from build123d import *

# Parameters (mm, degrees)
PAD011_DEPTH           = 3.5
POCKET_DEPTH           = 1
SKETCH_W               = 3
SKETCH_H               = 7
POCKET024_DEPTH        = 3.501
LINEARPATTERN001_COUNT = 3
LINEARPATTERN001_PITCH = 20


with BuildPart() as part:
    # Sketch030 (on Face1 of Binder) → Pad011 (new body)
    with BuildSketch(Plane(origin=(0, 0, -1.5), x_dir=(1, 0, 0), z_dir=(0, 0, -1))):
        Polygon((17.648, -218.84), (19.648, -220.84), (105.648, -220.84), (107.648, -218.84), (107.648, -139.715), (105.648, -137.715), (107.648, -135.715), (107.648, -56.59), (105.648, -54.59), (19.648, -54.59), (17.648, -56.59), (17.648, -135.715), (19.648, -137.715), (17.648, -139.715), align=None)
    extrude(amount=-PAD011_DEPTH)

    # Sketch034 (on Face4 of Pad011) → Pocket (cut)
    with BuildSketch(Plane.XY.offset(2)):
        Polygon((19.523, 137.84), (62.523, 137.84), (62.523, 220.84), (62.773, 220.84), (62.773, 137.84), (105.773, 137.84), (105.773, 137.59), (62.773, 137.59), (62.773, 54.59), (62.523, 54.59), (62.523, 137.59), (19.523, 137.59), align=None)
    extrude(amount=-POCKET_DEPTH, mode=Mode.SUBTRACT)

    # Sketch (on Face4 of Clone001) → Pocket024 (cut, through all)
    with BuildSketch(Plane.XY.offset(2)):
        with Locations((42.648, 137.715)):
            Rectangle(SKETCH_W, SKETCH_H)
        Polygon((40.198, 152.615), (43.098, 152.615), (43.098, 151.165), (44.548, 151.165), (44.548, 148.265), (43.098, 148.265), (43.098, 146.815), (40.198, 146.815), (40.198, 148.265), (38.748, 148.265), (38.748, 151.165), (40.198, 151.165), align=None)
        Polygon((40.198, 122.815), (43.098, 122.815), (43.098, 124.265), (44.548, 124.265), (44.548, 127.165), (43.098, 127.165), (43.098, 128.615), (40.198, 128.615), (40.198, 127.165), (38.748, 127.165), (38.748, 124.265), (40.198, 124.265), align=None)
    pocket024 = extrude(amount=-POCKET024_DEPTH, mode=Mode.SUBTRACT)

    # LinearPattern001: Pocket024 ×3
    with Locations(*[(i * LINEARPATTERN001_PITCH, 0, 0) for i in range(1, LINEARPATTERN001_COUNT)]):
        add(pocket024, mode=Mode.SUBTRACT)


with BuildPart() as part_1:
    # Body010 placement: moved
    add(part.part.moved(Location((204.403, 0, 0))))


solid = part_1.part
The model under review builds one solid part; all positions refer to its coordinate system, in mm. A direction names the side the tool comes from. Round coordinates to 2 decimals unless told otherwise and drop trailing zeros. Write item = value, one per line. Start each with the question number.
Item 1: For line 1 along Y through (x, z) = (259.5, 1.1); line 2 along X through (y, z) = (89.5, 1.1); line 3 along X through (y, z) = (137, -0.6), list the stretches that pass through material, from the lowest coordinate up.
Item 2: For faces 1 (the face through (289, 96, 2)), 2 (the face through (247, 141.215, 0)), list the 3-axis set-ups (+Z, -Z, +X, -X, +Y, -Y) from which the entire face can be reached by the end or side of a thin tool; tool diameter is ignored.
Item 3: Mouldability with a two-part tool opening along X and no side actions: class faces 3 (the face through (266, 152.615, 0)), 4 (the face through (312.051, 180, 0)), 5 (the face through (289, 179, 2)) as released by +X, released by -X, zero draft, split by the parting line, or undercut.
Item 4: Consider section A-A on z = -0.15. Count the separate pieces of the cut face and the enclosed holes in it, plus the area to 3 significant figures.
Conclusion:
q1.line_1 = 54.59 to 137.59, 137.84 to 220.84
q1.line_2 = 222.05 to 266.93, 267.18 to 312.05
q1.line_3 = 223.34 to 245.55, 248.55 to 265.55, 268.55 to 285.55, 288.55 to 310.77
q2.face_1 = +Z, +X, -X, +Y, -Y
q2.face_2 = +Z, -Z
q3.face_3 = undercut
q3.face_4 = released by +X
q3.face_5 = zero draft
q4.separate_pieces = 1
q4.enclosed_holes = 9
q4.area = 14,700 mm2
